Build history of the part. All positions in model axes, mm. Face numbers are marked on the shaded views. A direction names the side the tool comes from. Round coordinates to 2 decimals unless told otherwise and drop trailing zeros. Write each loop counter-clockwise with the first axis right and the second up, starting at its lowest first coordinate (ties: lowest second). Pieces come first, ordered by that corner, then holes.
from build123d import *

# Parameters (mm, degrees)
F3_DEPTH = 1.651
F4_DEPTH = 1.27
F5_W     = 43.18
F5_H     = 30.902041302
F6_DEPTH = 2


with BuildPart() as f3:
    # F2 (on face) → F3 (new body)
    with BuildSketch(Plane.XY):
        with BuildLine():
            Line((15.24, 32.0904812722), (-12.7, 32.0904812722))
            ThreePointArc((-12.7, 32.0904812722), (-14.4960512242, 31.3465324964), (-15.24, 29.5504812722))
            Line((-15.24, 29.5504812722), (-15.24, 13.8884399702))
            ThreePointArc((-15.24, 13.8884399702), (-14.4960512242, 12.092388746), (-12.7, 11.3484399702))
            Line((-12.7, 11.3484399702), (15.24, 11.3484399702))
            ThreePointArc((15.24, 11.3484399702), (17.0360512242, 12.092388746), (17.78, 13.8884399702))
            Line((17.78, 13.8884399702), (17.78, 29.5504812722))
            ThreePointArc((17.78, 29.5504812722), (17.0360512242, 31.3465324964), (15.24, 32.0904812722))
        make_face()
    extrude(amount=-F3_DEPTH)

    # F1 (on face) → F4 (join)
    with BuildSketch(Plane.XY):
        Polygon((-5.502041302, 24.4704812722), (-11.0040826039, 29.9725225741), (-11.0040826039, 18.9684399702), (-5.502041302, 13.4663986682), (5.502041302, 13.4663986682), (0, 18.9684399702), (-5.502041302, 18.9684399702), align=None)
        Polygon((5.502041302, 29.9725225741), (-5.502041302, 29.9725225741), (0, 24.4704812722), (5.502041302, 24.4704812722), (5.502041302, 18.9684399702), (11.0040826039, 13.245652739), (16.5061239059, 13.245652739), (11.0040826039, 18.9684399702), (11.0040826039, 24.4704812722), align=None)
    extrude(amount=F4_DEPTH)

    # F5 (on face) → F6 (join)
    with BuildSketch(Plane(origin=(0, 0, -1.651), x_dir=(1, 0, 0), z_dir=(0, 0, -1))):
        with Locations((1.27, -21.7194606212)):
            Rectangle(F5_W, F5_H)
    extrude(amount=F6_DEPTH)


solid = f3.part
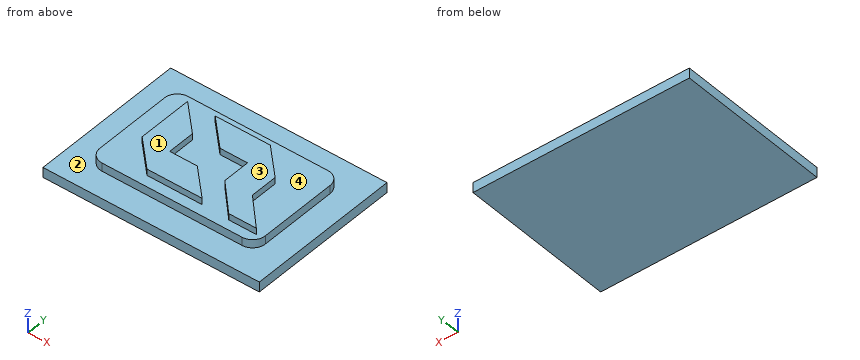
1) Pin check, flat tips, straight feed: pin 1 Ø0.6 at (x, z) = (4, 0.5) entering from -Y; pin 2 Ø0.6 at (y, z) = (21.5, 0.5) entering from +X; pin 3 Ø1.3 at (x, z) = (3, -0.5) entering from +Y. Stop position of each tip, or through.
Results:
pin 1: stops at y = 13.47
pin 2: stops at x = 11
pin 3: stops at y = 32.09
2) Slice it at A-A (z = -0.85). Write the cut outline in (x, y), plus the area to 3 significant figures.
Results:
outline: (-15.24, 13.89) arc R2.54 ccw to (-12.7, 11.35) - (15.24, 11.35) arc R2.54 ccw to (17.78, 13.89) - (17.78, 29.55) arc R2.54 ccw to (15.24, 32.09) - (-12.7, 32.09) arc R2.54 ccw to (-15.24, 29.55) - close
area: 679 mm2
3) Slice it at D-D (x = -2.5). Write the cut outline in (y, z).
Results:
outline: (6.27, -3.65) - (37.17, -3.65) - (37.17, -1.65) - (32.09, -1.65) - (32.09, 0) - (29.97, 0) - (29.97, 1.27) - (26.97, 1.27) - (26.97, 0) - (18.97, 0) - (18.97, 1.27) - (13.47, 1.27) - (13.47, 0) - (11.35, 0) - (11.35, -1.65) - (6.27, -1.65) - close
4) Wall check: L1, parallel to X at y = 22, z = 0.15; L2, parallel to X at y = 19.5, z = -0.75; L3, parallel to Z at x = 21.5, y = 21. Give the ranges that are in metal, low to high.
Results:
L1: x = -11 to -5.5, 5.5 to 11
L2: x = -15.24 to 17.78
L3: z = -3.65 to -1.65
5) Slice it at C-C (x = -14.5). Write the cut outline in (y, z), plus the area to 3 significant figures.
Results:
outline: (6.27, -3.65) - (37.17, -3.65) - (37.17, -1.65) - (31.34, -1.65) - (31.34, 0) - (12.1, 0) - (12.1, -1.65) - (6.27, -1.65) - close
area: 93.6 mm2
6) Mould opens along X. For the marked faces 3 and 4 say: released by +X, released by -X, zero draft, split by the parting line, or undercut.
Results:
face 3: zero draft
face 4: undercut
7) Which spindle directions (+Z, -Z, +X, -X, +Y, -Y) get a long thin tool onto all of the face, cutting with end or side? Do the marked faces 1 and 2. Say none if no direction does.
Results:
face 1: +Z, +X, -X, +Y, -Y
face 2: +Z
8) Slice it at B-B (y = 22). Write the cut outline in (x, z).
Results:
outline: (-20.32, -3.65) - (22.86, -3.65) - (22.86, -1.65) - (17.78, -1.65) - (17.78, 0) - (11, 0) - (11, 1.27) - (5.5, 1.27) - (5.5, 0) - (-5.5, 0) - (-5.5, 1.27) - (-11, 1.27) - (-11, 0) - (-15.24, 0) - (-15.24, -1.65) - (-20.32, -1.65) - close
